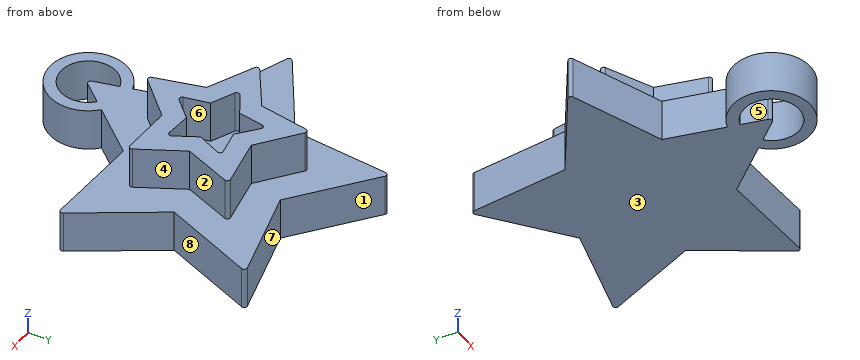
```python
from build123d import *

# Parameters (mm, degrees)
F1_DEPTH  = 7.62
F3_DEPTH  = 7.62
F5_DEPTH  = 7.62
F8_DEPTH  = 7.62
F10_DEPTH = 7.62
F12_DEPTH = 7.62


# Not quite as in the source:
# - a feature names something its author has since deleted; it is built from what else it names


with BuildPart() as f1:
    # F0 (on Top) → F1 (new body)
    with BuildSketch(Plane.XY):
        with BuildLine():
            Line((5.2457718421, 22.65034753), (-16.6286527122, 42.176813326))
            ThreePointArc((-16.6286527122, 42.176813326), (-17.1554325452, 42.2695789476), (-17.4732486395, 41.8393518177))
            Line((-17.4732486395, 41.8393518177), (-19.9207279669, 11.9883678087))
            Line((-19.9207279669, 11.9883678087), (-45.2510694319, -2.7814364328))
            ThreePointArc((-45.2510694319, -2.7814364328), (-45.5020787015, -3.2537676721), (-45.1911189603, -3.6889762341))
            Line((-45.1911189603, -3.6889762341), (-17.5574588063, -15.2411287545))
            Line((-17.5574588063, -15.2411287545), (-11.338046224, -43.895835579))
            ThreePointArc((-11.338046224, -43.895835579), (-10.9663986511, -44.2805179605), (-10.4563988677, -44.1192645141))
            Line((-10.4563988677, -44.1192645141), (9.0696216685, -21.4079034059))
            Line((9.0696216685, -21.4079034059), (38.2437714994, -24.3476819196))
            ThreePointArc((38.2437714994, -24.3476819196), (38.724471601, -24.1130974669), (38.7287090602, -23.5782287943))
            Line((38.7287090602, -23.5782287943), (23.1627932625, 2.0103168218))
            Line((23.1627932625, 2.0103168218), (34.9739968686, 28.8481406054))
            ThreePointArc((34.9739968686, 28.8481406054), (34.8994382969, 29.3778041519), (34.3920574073, 29.5471177247))
            Line((34.3920574073, 29.5471177247), (5.2457718421, 22.65034753))
        make_face()
    extrude(amount=F1_DEPTH)

    # F2 (on face) → F3 (join)
    with BuildSketch(Plane.XY.offset(7.62)):
        with BuildLine():
            Line((-10.7096949682, 24.1632334685), (-12.0244422161, 7.2461689852))
            Line((-12.0244422161, 7.2461689852), (-26.367554987, -1.8197422817))
            ThreePointArc((-26.367554987, -1.8197422817), (-26.6022582168, -2.2927760227), (-26.2900783947, -2.7186754062))
            Line((-26.2900783947, -2.7186754062), (-10.6072732242, -9.1967347639))
            Line((-10.6072732242, -9.1967347639), (-6.4173448361, -25.6393662796))
            ThreePointArc((-6.4173448361, -25.6393662796), (-6.0399903009, -26.0087577805), (-5.5384670466, -25.8434672739))
            Line((-5.5384670466, -25.8434672739), (5.4687868356, -12.9300636548))
            Line((5.4687868356, -12.9300636548), (22.4014177608, -14.026257529))
            ThreePointArc((22.4014177608, -14.026257529), (22.8693389191, -13.7815202908), (22.8671175143, -13.2534657562))
            Line((22.8671175143, -13.2534657562), (13.9871693659, 1.2055159485))
            Line((13.9871693659, 1.2055159485), (20.2621824084, 16.9706623917))
            ThreePointArc((20.2621824084, 16.9706623917), (20.1740190532, 17.4913098242), (19.6711228952, 17.6523749678))
            Line((19.6711228952, 17.6523749678), (3.1757592389, 13.675113485))
            Line((3.1757592389, 13.675113485), (-9.8787003461, 24.5147036987))
            ThreePointArc((-9.8787003461, 24.5147036987), (-10.4011094545, 24.5917442699), (-10.7096949682, 24.1632334685))
        make_face()
    extrude(amount=F3_DEPTH)

    # F4 (on face) → F5 (join)
    with BuildSketch(Plane.XY.offset(15.24)):
        with BuildLine():
            ThreePointArc((-4.7045563215, 13.3742015157), (-5.2088793669, 13.454135563), (-5.5278964741, 13.0554385961))
            Line((-5.5278964741, 13.0554385961), (-6.8203753298, 4.4014452639))
            Line((-6.8203753298, 4.4014452639), (-14.1734093561, -0.3414433913))
            ThreePointArc((-14.1734093561, -0.3414433913), (-14.4052755444, -0.7963821309), (-14.1246739036, -1.2229895678))
            Line((-14.1246739036, -1.2229895678), (-6.2936350842, -5.1264410146))
            Line((-6.2936350842, -5.1264410146), (-4.0550923971, -13.5852251368))
            ThreePointArc((-4.0550923971, -13.5852251368), (-3.6940705368, -13.946326788), (-3.2016320784, -13.811287717))
            Line((-3.2016320784, -13.811287717), (2.9306949349, -7.5697600522))
            Line((2.9306949349, -7.5697600522), (11.6672244272, -8.0546874881))
            ThreePointArc((11.6672244272, -8.0546874881), (12.1222143958, -7.8229218423), (12.1459564597, -7.3128556696))
            Line((12.1459564597, -7.3128556696), (8.1049041646, 0.4480720157))
            Line((8.1049041646, 0.4480720157), (11.2658336475, 8.6071545004))
            ThreePointArc((11.2658336475, 8.6071545004), (11.1860110523, 9.1114951981), (10.7082459963, 9.2916943583))
            Line((10.7082459963, 9.2916943583), (2.0784113144, 7.8466837873))
            Line((2.0784113144, 7.8466837873), (-4.7045563215, 13.3742015157))
        make_face()
    extrude(amount=F5_DEPTH)

    # F8 (cut): a face of the model
    f8_faces = [f1.faces().sort_by_distance(p)[0] for p in [
        (0, 0, 0),
    ]]
    extrude(f8_faces, amount=-F8_DEPTH, mode=Mode.SUBTRACT)

    # F9 (on face) → F10 (cut)
    with BuildSketch(Plane.XY.offset(22.86)):
        with BuildLine():
            ThreePointArc((-2.1197789922, 7.0861071574), (-2.6315872512, 7.1830271414), (-2.9596514058, 6.77840993))
            Line((-2.9596514058, 6.77840993), (-3.5885418896, 2.4094997361))
            Line((-3.5885418896, 2.4094997361), (-7.3943361202, 0.173697912))
            ThreePointArc((-7.3943361202, 0.173697912), (-7.6446699524, -0.2831107457), (-7.3612335158, -0.7201518922))
            Line((-7.3612335158, -0.7201518922), (-3.400490854, -2.6683297817))
            Line((-3.400490854, -2.6683297817), (-2.4501720543, -6.9787559441))
            ThreePointArc((-2.4501720543, -6.9787559441), (-2.0930786121, -7.3579992049), (-1.5898411061, -7.2234882764))
            Line((-1.5898411061, -7.2234882764), (1.4869229634, -4.0586182344))
            Line((1.4869229634, -4.0586182344), (5.8800465123, -4.4868062846))
            ThreePointArc((5.8800465123, -4.4868062846), (6.351076229, -4.2643828521), (6.3786576755, -3.7442093799))
            Line((6.3786576755, -3.7442093799), (4.319459784, 0.1599657655))
            Line((4.319459784, 0.1599657655), (6.0842406543, 4.2057571592))
            ThreePointArc((6.0842406543, 4.2057571592), (6.0182595868, 4.7224656612), (5.5320683522, 4.9094396186))
            Line((5.5320683522, 4.9094396186), (1.1826499962, 4.1574825145))
            Line((1.1826499962, 4.1574825145), (-2.1197789922, 7.0861071574))
        make_face()
    extrude(amount=-F10_DEPTH, mode=Mode.SUBTRACT)

    # F11 (on face) → F12 (join)
    with BuildSketch(Plane(origin=(0, 0, 7.62), x_dir=(1, 0, 0), z_dir=(0, 0, -1))):
        with BuildLine():
            Line((-2.6220134118, 22.4219651148), (-1.3098667841, 20.8825912445))
            ThreePointArc((-1.3098667841, 20.8825912445), (-7.6178176155, 32.8030283673), (-8.0269681328, 19.3226848722))
            Line((-8.0269681328, 19.3226848722), (-7.5274974689, 21.282768988))
            ThreePointArc((-7.5274974689, 21.282768988), (-7.1607580244, 30.8348874257), (-2.6220134118, 22.4219651148))
        make_face()
    extrude(amount=-F12_DEPTH)


solid = f1.part
```
Design review of the part built by this model. Coordinates are the model's own, in mm. Face numbers are marked on the shaded views. A direction names the side the tool comes from. Round coordinates to 2 decimals unless told otherwise and drop trailing zeros. Write each loop counter-clockwise with the first axis right and the second up, starting at its lowest first coordinate (ties: lowest second). Pieces come first, ordered by that corner, then holes. Notation, with made-up numbers: (-12, 43) -> (7, 43) arc R10 ccw to (7, 49) -> close; hole circle Ø1 at (26, -13.75). An arc over 180 degrees is marked (long way). Write item = value, one per line. Start each with the question number.
1) Take a section at C-C, the plane x = 17.5. State the section outline as (y, z) points, plus the area to 3 significant figures.
2) Wall thickness on probe 1 along Z at (x, y) = (13, -2); probe 2 along X at (y, z) = (-3.5, 19.75); probe 3 along X at (y, z) = (-2, 16.75): over which ranges is each line inside the solid? List them lowest first. Write a range as from..to.
3) Take a section at B-B, the plane y = -24. State the section outline as (x, z) points, plus the area to 3 significant figures.
4) Clearance check with flat-ended pins moving along their axes: pin 1 (2 mm diameter, centred on x = -16.5, z = 10.5, fed in from -Y); pin 2 (5 mm diameter, centred on x = -19.5, z = 12.5, fed in from -Y); pin 3 (13 mm diameter, centred on x = -6.04, y = -26.01, fed in from +Z). State where each tip first meets the part, or that it passes through.
5) Mouldability with a two-part tool opening along Y and no side actions: class the marked faces 1, 2 and 3 as +Y half, -Y half, draft (parallel to the pull), parting line (faces both ways), or undercut.
6) Take a section at D-D, the plane y = 15.5. State the section outline as (x, z) points.
7) Tool access review of the marked faces 4, 5, 6, 7 and 8: name each direction out of +Z, -Z, +X, -X, +Y, -Y from which nothing blocks a thin tool from reaching the whole face with its end or side.
Results list:
q1.outline = (-13.71, 7.62) -> (-4.51, 7.62) -> (-4.51, 15.24) -> (-13.71, 15.24) -> close; (10.03, 7.62) -> (17.13, 7.62) -> (17.13, 15.24) -> (10.03, 15.24) -> close
q1.area = 124 mm²
q2.probe_1 = 7.62..15.24
q2.probe_2 = -9.56..-3.22, 6.25..10.16
q2.probe_3 = -12.57..-4.76, 5.46..9.38
q3.outline = (-12.72, 7.62) -> (-10.57, 7.62) -> (-10.57, 15.24) -> (-12.72, 15.24) -> close; (-6.84, 7.62) -> (-3.97, 7.62) -> (-3.97, 15.24) -> (-6.84, 15.24) -> close; (-1.51, 7.62) -> (0.64, 7.62) -> (0.64, 15.24) -> (-1.51, 15.24) -> close
q3.area = 54.6 mm²
q4.pin_1 = -7.18
q4.pin_2 = -6.56
q4.pin_3 = 15.24
q5.face_1 = +Y half
q5.face_2 = undercut
q5.face_3 = draft
q6.outline = (-11.38, 7.62) -> (0.98, 7.62) -> (0.98, 15.24) -> (-11.38, 15.24) -> close; (10.74, 7.62) -> (19.68, 7.62) -> (19.68, 15.24) -> (10.74, 15.24) -> close
q7.face_4 = +Z, +X
q7.face_5 = +Z, -Z
q7.face_6 = +Z
q7.face_7 = +Z, -Z, +Y
q7.face_8 = +Z, -Z, +X
